Build history of the part. All positions in model axes, mm. A direction names the side the tool comes from. Round coordinates to 2 decimals unless told otherwise and drop trailing zeros. Write each loop counter-clockwise with the first axis right and the second up, starting at its lowest first coordinate (ties: lowest second). Pieces come first, ordered by that corner, then holes. Notation, with made-up numbers: (12, 76.5) -> (26, 76.5) arc R13 cw to (26, 97.5) -> close; hole circle Ø10 at (37, -21). An arc over 180 degrees is marked (long way). Answer in a Markdown table with one row per item. Add a question column.
from build123d import *

# Parameters (mm, degrees)
SKETCH1_R               = 1
BOSS_EXTRUDE1_DEPTH     = 30
SKETCH3_R               = 1
BOSS_EXTRUDE2_DEPTH     = 3
CUT_EXTRUDE1_REACH      = 70.622
CUT_EXTRUDE1_END_RADIUS = 9.5
SKETCH4_R               = 5


with BuildPart() as part:
    # Sketch1 → Boss-Extrude1 (new body)
    with BuildSketch(Plane.XY):
        with BuildLine():
            Line((141, -22), (87, -22))
            ThreePointArc((87, -22), (86.292893219, -21.707106781), (86, -21))
            Line((86, -21), (86, -2))
            ThreePointArc((86, -2), (86.292893219, -1.292893219), (87, -1))
            Line((87, -1), (141, -1))
            ThreePointArc((141, -1), (141.707106781, -1.292893219), (142, -2))
            Line((142, -2), (142, -21))
            ThreePointArc((142, -21), (141.707106781, -21.707106781), (141, -22))
        make_face()
        with Locations((140, -3)):
            Circle(SKETCH1_R, mode=Mode.SUBTRACT)
        with Locations((88, -3)):
            Circle(SKETCH1_R, mode=Mode.SUBTRACT)
        with Locations((88, -20)):
            Circle(SKETCH1_R, mode=Mode.SUBTRACT)
        with Locations((140, -20)):
            Circle(SKETCH1_R, mode=Mode.SUBTRACT)
        with BuildLine():
            Line((131.5, -21), (96.5, -21))
            ThreePointArc((96.5, -21), (87, -11.5), (96.5, -2))
            Line((96.5, -2), (131.5, -2))
            ThreePointArc((131.5, -2), (141, -11.5), (131.5, -21))
        make_face(mode=Mode.SUBTRACT)
    extrude(amount=BOSS_EXTRUDE1_DEPTH)

    # Sketch3 → Boss-Extrude2 (add)
    with BuildSketch(Plane.XY.offset(30)):
        with BuildLine():
            Line((86, -2), (86, -21))
            ThreePointArc((86, -21), (86.292893219, -21.707106781), (87, -22))
            Line((87, -22), (141, -22))
            ThreePointArc((141, -22), (141.707106781, -21.707106781), (142, -21))
            Line((142, -21), (142, -2))
            ThreePointArc((142, -2), (141.707106781, -1.292893219), (141, -1))
            Line((141, -1), (87, -1))
            ThreePointArc((87, -1), (86.292893219, -1.292893219), (86, -2))
        make_face()
        with Locations((88, -3)):
            Circle(SKETCH3_R, mode=Mode.SUBTRACT)
        with Locations((88, -20)):
            Circle(SKETCH3_R, mode=Mode.SUBTRACT)
        with Locations((140, -20)):
            Circle(SKETCH3_R, mode=Mode.SUBTRACT)
        with Locations((140, -3)):
            Circle(SKETCH3_R, mode=Mode.SUBTRACT)
    extrude(amount=BOSS_EXTRUDE2_DEPTH)

    # Cut-Extrude1: up to this cylinder (the profile starts outside it)
    cut_extrude1_end = Plane(origin=(96.5, -11.5, 23), z_dir=(0, 0, -1)) * Cylinder(CUT_EXTRUDE1_END_RADIUS, 161.244, mode=Mode.PRIVATE)
    # Sketch4 → Cut-Extrude1 (cut, up to the surface)
    with BuildSketch(Plane.ZY.offset(-86), mode=Mode.PRIVATE) as cut_extrude1_sk1:
        with Locations((23, -11.5)):
            Circle(SKETCH4_R)
    cut_extrude1_tool1 = extrude(cut_extrude1_sk1.sketch, amount=-CUT_EXTRUDE1_REACH, mode=Mode.PRIVATE) - cut_extrude1_end
    add(cut_extrude1_tool1.solids().sort_by_distance((86, -11.5, 23))[0], mode=Mode.SUBTRACT)


solid = part.part
(1) Saw through at D-D (y = -3). List the corners of the cut face in (x, z), plus the area to 3 significant figures.
(2) Saw through at B-B (z = 14). List the corners of the cut face in (x, y), plus the area to 3 significant figures.
(3) Saw through at C-C (x = 140). List the corners of the cut face in (y, z).
(4) Mould opens along X. For faces 4 (the face through (142, -12, 16)), 5 (the face through (86, -11, 16)), 6 (the face through (114, -21, 15)), 7 (the face through (114, -1, 16)) say: pulls with the +X half, pulls with the -X half, needs draft (parallel to the pull), parting line crosses it, or undercut.
(5) Drop flat-ended pins along their axis: P1, Ø2.5, axis at x = 88, y = -20, coming from the +Z side; P2, Ø8, axis at y = -11.5, z = 23, coming from the -X side; P3, Ø9.5, axis at x = 116.5, y = -12, coming from the -Z side. Give the stop position or say it passes through.
(6) Saw through at A-A (y = -11.5). List the corners of the cut face in (x, z).
(7) Which spindle directions (+Z, -Z, +X, -X, +Y, -Y) get a long thin tool onto all of the face, cutting with end or side? Do faces 1 (the face through (139.2, -3.6, 16.3)), 2 (the face through (114, -2, 15)), 3 (the face through (86.93, -16.38, 21.92)). Say none if no direction does.
(8) Probe line 1 along Y through (x, z) = (111, 12); line 2 along Y through (x, z) = (140, 11.5); line 3 along Z through (x, y) = (94, -12). List the from-to ranges inside material, lowest first.
Answer sheet:
| question | item | result |
|---|---|---|
| 1 | outline | (86, 0) -> (87, 0) -> (87, 33) -> (86, 33) -> close; (89, 0) -> (92.26, 0) -> (92.26, 30) -> (135.74, 30) -> (135.74, 0) -> (139, 0) -> (139, 33) -> (89, 33) -> close; (141, 0) -> (142, 0) -> (142, 33) -> (141, 33) -> close |
| 1 | area | 411 mm² |
| 2 | outline | (86, -21) arc R1 ccw to (87, -22) -> (141, -22) arc R1 ccw to (142, -21) -> (142, -2) arc R1 ccw to (141, -1) -> (87, -1) arc R1 ccw to (86, -2) -> close; hole circle Ø2 at (88, -20); hole circle Ø2 at (88, -3); hole (96.5, -21) -> (131.5, -21) arc R9.5 ccw to (131.5, -2) -> (96.5, -2) arc R9.5 ccw to start; hole circle Ø2 at (140, -20); hole circle Ø2 at (140, -3) |
| 2 | area | 214 mm² |
| 3 | outline | (-22, 0) -> (-21, 0) -> (-21, 33) -> (-22, 33) -> close; (-19, 0) -> (-15.74, 0) -> (-15.74, 30) -> (-7.26, 30) -> (-7.26, 0) -> (-4, 0) -> (-4, 33) -> (-19, 33) -> close; (-2, 0) -> (-1, 0) -> (-1, 33) -> (-2, 33) -> close |
| 4 | face 4 | pulls with the +X half |
| 4 | face 5 | pulls with the -X half |
| 4 | face 6 | undercut |
| 4 | face 7 | needs draft |
| 5 | P1 | stops at z = 33 |
| 5 | P2 | stops at x = 140.12 |
| 5 | P3 | stops at z = 30 |
| 6 | outline | (86, 0) -> (87, 0) -> (87, 18) -> (86, 18) -> close; (86, 28) -> (87, 28) -> (87, 30) -> (141, 30) -> (141, 0) -> (142, 0) -> (142, 33) -> (86, 33) -> close |
| 7 | face 1 | +Z, -Z |
| 7 | face 2 | -Z |
| 7 | face 3 | -X |
| 8 | line 1 | y = -22 to -21, -2 to -1 |
| 8 | line 2 | y = -22 to -21, -19 to -15.74, -7.26 to -4, -2 to -1 |
| 8 | line 3 | z = 30 to 33 |
